Part print with two shaded views. Sizes in mm from the minimum x, y, z corner. A direction names the side the tool comes from. Round coordinates to 2 decimals unless told otherwise and drop trailing zeros. Loops run counter-clockwise (first coordinate to the right, second up) from the corner with the lowest first, then second, coordinate; pieces in that order, holes last. Notation, with made-up numbers: (76, -23) - (84, -23) arc R27 ccw to (84, -4) - close; hole circle Ø10 at (61.25, 8.25). An arc over 180 degrees is marked (long way). Write each question's results on one line, items separated by ' | '. Start each with the question number.
(1) Cut at C-C, the plane y = 0.5. List the corners of the cut face in (x, z).
(2) Tool access for the marked faces 1 and 2: list every direction of +Z, -Z, +X, -X, +Y, -Y with a clear straight run to the whole face (end or side of a thin tool).
(3) Cut at D-D, the plane x = 1.75. List the corners of the cut face in (y, z).
(4) Flat gauge pins, fed straight in: P1, Ø1.5, axis at y = 1, z = 10, coming from the -X side; P2, Ø6, axis at x = 6.5, z = 6.5, coming from the +Y side; P3, Ø1, axis at x = 11.5, y = 3, coming from the -Z side (1 decimal). Where does each tip first touch, or does it go through?
(5) Drill centre lines: L1, parallel to Y at x = 3, z = 1.25; L2, parallel to Z at x = 8.5, y = 3.65 (1 decimal); L3, parallel to X at y = 0.9, z = 6.25 (1 decimal). Where is each one in solid material? Low to high.
(6) Mould opens along X. For the marked faces 3, 4 and 5 say: released by +X, released by -X, zero draft, split by the parting line, or undercut.
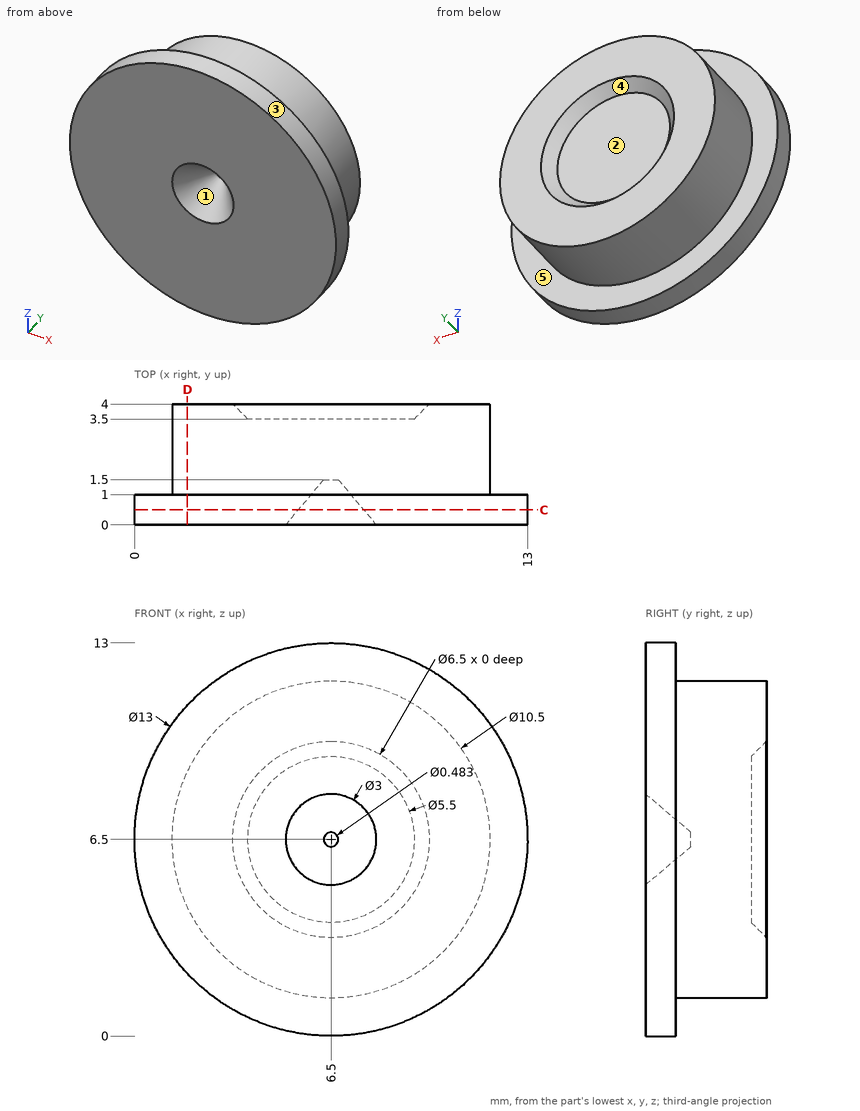
A:
1) outline: circle Ø13 at (6.5, 6.5); hole circle Ø2.16 at (6.5, 6.5)
2) face 1: -Y | face 2: +Y
3) outline: (0, 2.06) - (1, 2.06) - (1, 4.26) - (4, 4.26) - (4, 8.74) - (1, 8.74) - (1, 10.94) - (0, 10.94) - close
4) P1: x = 0.61 | P2: y = 3.75 | P3: z = 3.8
5) L1: 0 to 1 | L2: 1.6 to 4.4, 8.6 to 11.4 | L3: 0 to 5.8, 7.2 to 13
6) face 3: split by the parting line | face 4: undercut | face 5: zero draft
